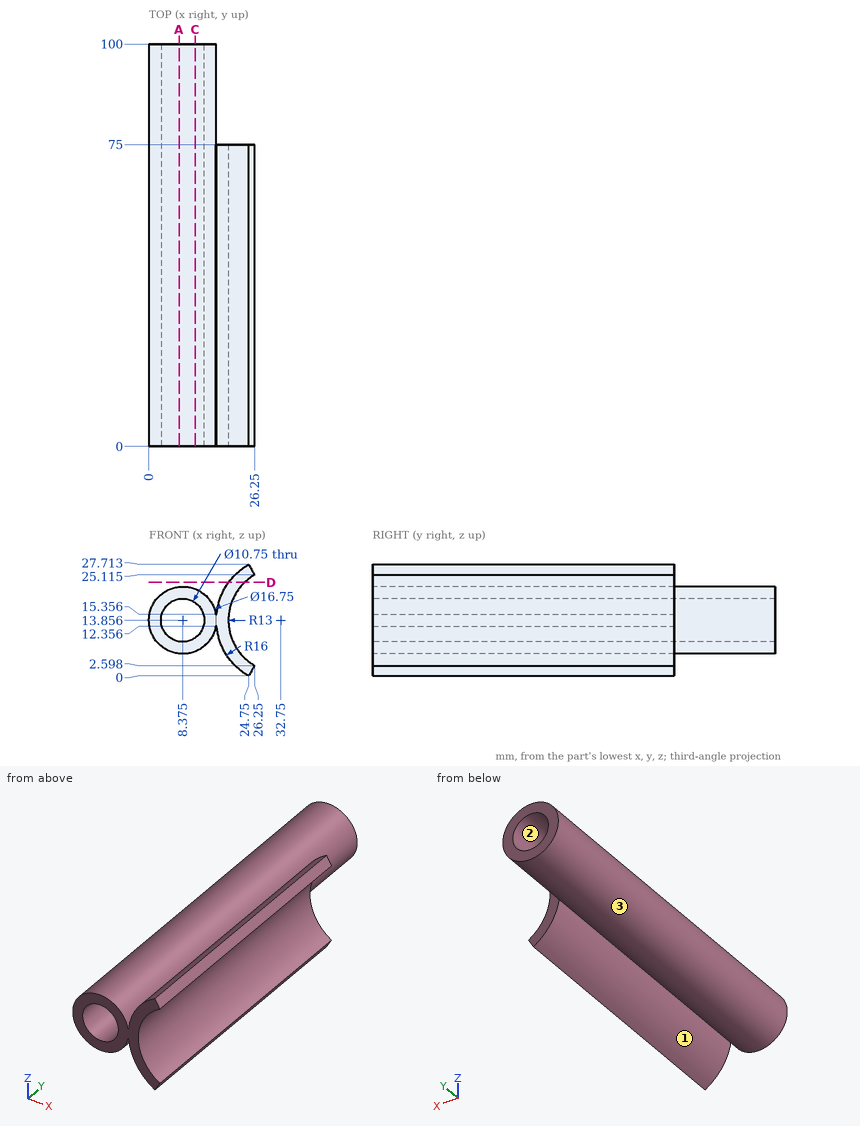
Input: dimensioned drawing with shaded views. Units: mm. Origin: part minimum x, y, z. Round coordinates to 2 decimals unless told otherwise and drop trailing zeros. Loops run counter-clockwise (first coordinate to the right, second up) from the corner with the lowest first, then second, coordinate; pieces in that order, holes last. Notation, with made-up numbers: (-34, 9.25) -> (-6, 9.25) arc R20 ccw to (-6, 14.25) -> close; hole circle Ø11 at (-34.75, 85.5). An arc over 180 degrees is marked (long way). Answer as a JSON object with one key per item and string values. Group by question number.
Q1. Section query A-A (x = 7.5). Output: boundary loops of the cut face in (y, z) (1 decimal).
Q2. Section query C-C (x = 11.5). Output: boundary loops of the cut face in (y, z).
Q3. Mould query, pull axis Z, two halves, no side actions, for the marked faces 1, 2 and 3. Classes: pulls with the +Z half, pulls with the -Z half, needs draft (parallel to the pull), parting line crosses it, or undercut.
Q4. Contact query for flat-ended pins moving along their axis: P1, Ø1, axis at x = 14.5, y = 13, coming from the -Z side; P2, Ø1, axis at y = 80.5, z = 3, coming from the +X side; P3, Ø5, axis at x = 17.5, z = 24, coming from the +Y side; P4, Ø1.5, axis at x = 19, y = 69.5, coming from the -Z side. Output: stop coordinate, or through.
Q5. Section query D-D (z = 23.25). Output: boundary loops of the cut face in (x, y).
Q6. Ray query, line 1 (Y direction, x = 17.5, z = 17.5); line 2 (X direction, y = 57.5, z = 15); line 3 (Z direction, x = 21.5, y = 6) (1 decimal). Return the intervals inside material, ascending. Write a range as from..to.
Completed:
{
 "1": {"outline": "(0, 5.5) -> (100, 5.5) -> (100, 8.6) -> (0, 8.6) -> close; (0, 19.2) -> (100, 19.2) -> (100, 22.2) -> (0, 22.2) -> close"},
 "2": {"outline": "(0, 6.09) -> (100, 6.09) -> (100, 9.48) -> (0, 9.48) -> close; (0, 18.23) -> (100, 18.23) -> (100, 21.63) -> (0, 21.63) -> close"},
 "3": {"face 1": "pulls with the -Z half", "face 2": "undercut", "face 3": "parting line crosses it"},
 "4": {"P1": "z = 7.65", "P2": "through", "P3": "y = 75", "P4": "z = 4.53"},
 "5": {"outline": "(19.8, 0) -> (23.76, 0) -> (23.76, 75) -> (19.8, 75) -> close"},
 "6": {"line 1": "0..75", "line 2": "0.08..3.12, 13.63..19.8", "line 3": "2.5..7.3, 20.4..25.2"}
}
